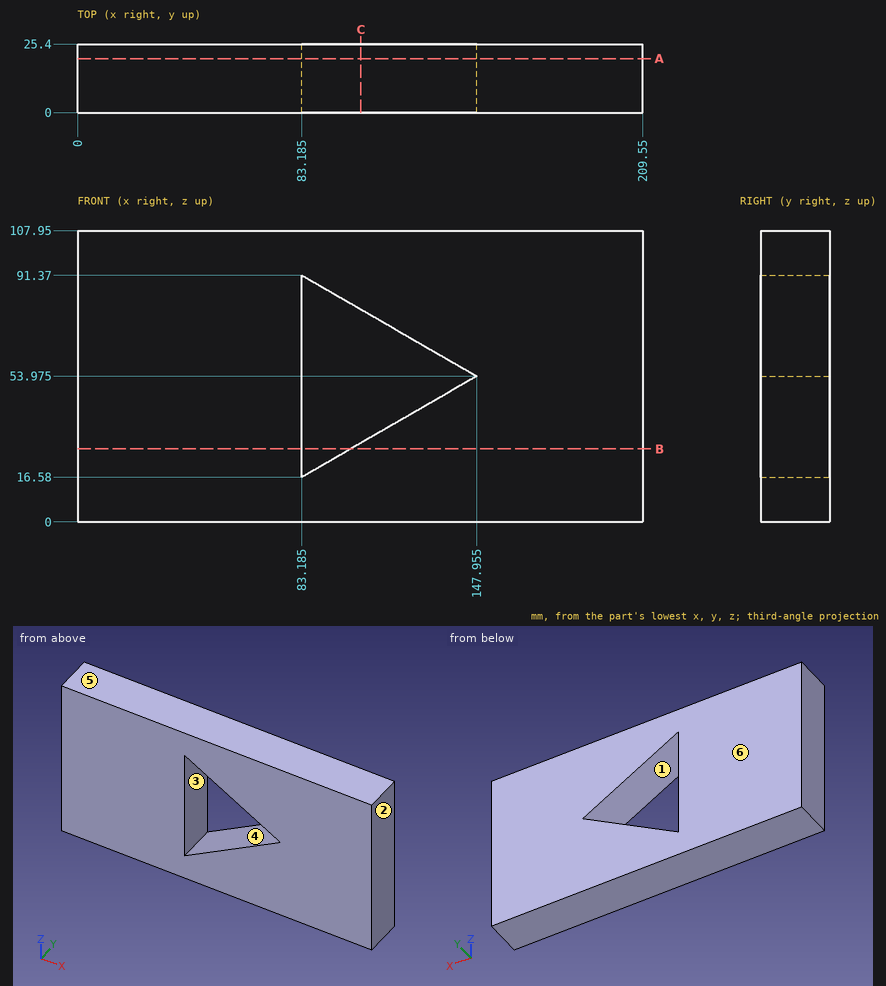
Input: dimensioned drawing with shaded views. Units: mm. Origin: part minimum x, y, z. A direction names the side the tool comes from. Coordinates: 2 decimals unless noted, no trailing zeros. Order: outer loops, then holes, each group sorted by start corner. A loop starts at its lowest first (then second) coordinate and runs counter-clockwise, first axis right, second up. Notation, with made-up numbers: (34.5, 24) - (51.5, 24) arc R8 cw to (51.5, 28) - close; hole circle Ø11 at (-21.5, 6). An arc over 180 degrees is marked (long way). Return JSON: item names as keys, results as strings. Group by question number.
1. Cut plane A-A (y = 20). Output: boundary loops of the cut face in (x, z) (3 decimals), plus the area to 3 significant figures.
2. Pin query (flat end, axial travel): pin 1 (3 mm diameter, centred on x = 144, y = 6.5, fed in from -Z). Return the tip coordinate at first contact, or that it passes through.
3. Cut plane C-C (x = 105). Output: boundary loops of the cut face in (y, z).
4. Set-up query: the marked faces 1 and 2. Return all of +Z, -Z, +X, -X, +Y, -Y with unobstructed straight access to the full face (end or side cutting, diameter ignored); none if empty.
5. Material intervals for line 1 along Z through (x, y) = (114, 9); line 2 along X through (y, z) = (3, 25.5) (3 decimals); line 3 along X through (y, z) = (13.5, 47.5) (3 decimals), sorted ascending. Write a range as [from, to].
6. Cut plane B-B (z = 27). Output: boundary loops of the cut face in (x, y) (3 decimals).
7. Pull-direction query (Z, two-part tool) for the marked faces 3, 4, 5 and 6; classes: pulls with the +Z half, pulls with the -Z half, needs draft (parallel to the pull), parting line crosses it, or undercut.
Resolved:
{
 "1": {"outline": "(0, 0) - (209.55, 0) - (209.55, 107.95) - (0, 107.95) - close; hole (83.185, 16.58) - (147.955, 53.975) - (83.185, 91.37) - close", "area": "20,200 mm²"},
 "2": {"pin 1": "stops at z = 0"},
 "3": {"outline": "(0, 0) - (25.4, 0) - (25.4, 29.17) - (0, 29.17) - close; (0, 78.78) - (25.4, 78.78) - (25.4, 107.95) - (0, 107.95) - close"},
 "4": {"face 1": "+Y, -Y", "face 2": "+Z, -Z, +X, +Y, -Y"},
 "5": {"line 1": "z = [0, 34.37], [73.58, 107.95]", "line 2": "x = [0, 83.185], [98.635, 209.55]", "line 3": "x = [0, 83.185], [136.74, 209.55]"},
 "6": {"outline": "(0, 0) - (83.185, 0) - (83.185, 25.4) - (0, 25.4) - close; (101.233, 0) - (209.55, 0) - (209.55, 25.4) - (101.233, 25.4) - close"},
 "7": {"face 3": "undercut", "face 4": "undercut", "face 5": "pulls with the +Z half", "face 6": "needs draft"}
}
